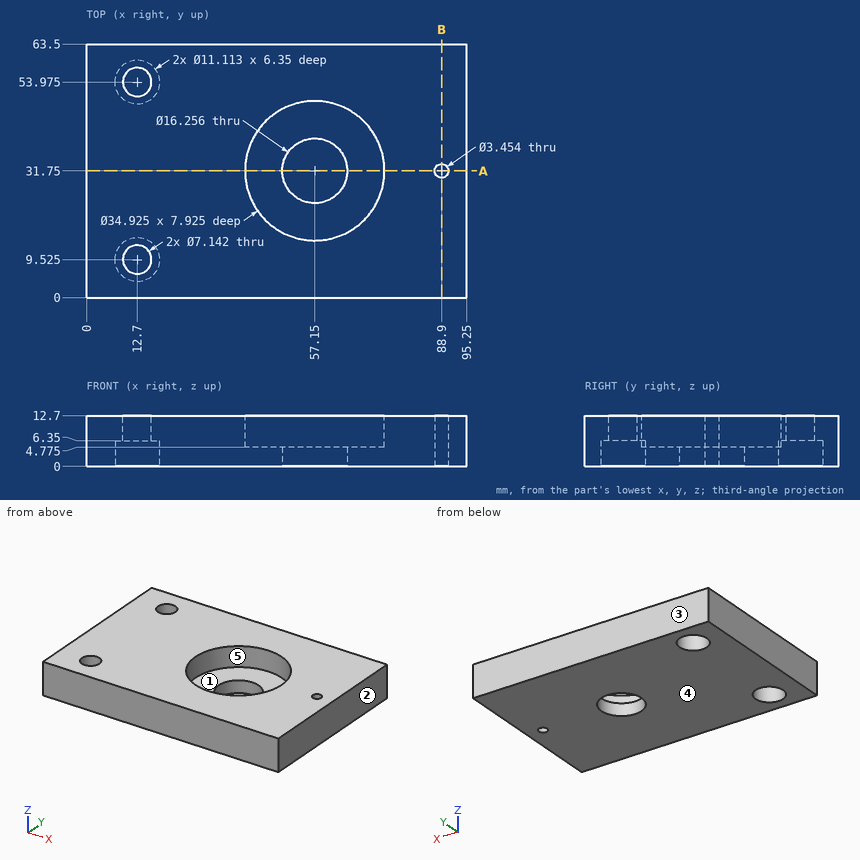
Design review of the part shown in the three views and the two pictorial views. Dimensions are in mm from the part's minimum x, y and z. A direction names the side the tool comes from. Round coordinates to 2 decimals unless told otherwise and drop trailing zeros. Write each loop counter-clockwise with the first axis right and the second up, starting at its lowest first coordinate (ties: lowest second). Pieces come first, ordered by that corner, then holes. Notation, with made-up numbers: (70.5, 40) - (121.5, 40) arc R13 ccw to (121.5, 53) - close; hole circle Ø1 at (-25, 81). An arc over 180 degrees is marked (long way). Write item = value, one per line. Start each with the question number.
1. Consider section A-A on y = 31.75. Give the number of separate pieces and of enclosed holes in the cut face.
2. Consider section B-B on x = 88.9. State the section outline as (y, z) points.
3. Draft analysis for pull direction Y (two halves, no side actions). For the marked faces 1, 2 and 3, state which applies: released by +Y, released by -Y, zero draft, split by the parting line, or undercut.
4. For the marked faces 4 and 5, list the 3-axis set-ups (+Z, -Z, +X, -X, +Y, -Y) from which the entire face can be reached by the end or side of a thin tool; tool diameter is ignored.
5. Wall thickness on L1, parallel to Y at x = 12.7, z = 4.25; L2, parallel to Y at x = 57.15, z = 1.2; L3, parallel to Y at x = 52, z = 6.75 (1 decimal): over which ranges is each line inside the solid? List them lowest first.
Evaluation:
q1.separate_pieces = 3
q1.enclosed_holes = 0
q2.outline = (0, 0) - (30.02, 0) - (30.02, 12.7) - (0, 12.7) - close; (33.48, 0) - (63.5, 0) - (63.5, 12.7) - (33.48, 12.7) - close
q3.face_1 = undercut
q3.face_2 = zero draft
q3.face_3 = released by +Y
q4.face_4 = -Z, +X, -X, +Y, -Y
q4.face_5 = +Z
q5.L1 = 0 to 3.97, 15.08 to 48.42, 59.53 to 63.5
q5.L2 = 0 to 23.62, 39.88 to 63.5
q5.L3 = 0 to 15.1, 48.4 to 63.5
